The listing builds one solid part. Answer for the finished solid, in the listing's coordinates (mm). A direction names the side the tool comes from. Coordinates: 2 decimals unless noted, no trailing zeros. Order: outer loops, then holes, each group sorted by start corner. A loop starts at its lowest first (then second) coordinate and runs counter-clockwise, first axis right, second up. Notation, with made-up numbers: (22, 53) -> (28, 53) arc R5 ccw to (28, 61) -> close; hole circle Ø4 at (-16, 20). An arc over 180 degrees is marked (long way). Answer in a Markdown table with one row per item. Add a question column.
```python
from build123d import *

# Parameters (mm, degrees)
F0_W     = 119.054884
F0_H     = 68.104512
F1_DEPTH = 25.4
F2_R     = 23.34143
F3_DEPTH = 47.244
F5_DEPTH = 32.512


with BuildPart() as f1:
    # F0 (on Top) → F1 (new body)
    with BuildSketch(Plane.XY):
        Rectangle(F0_W, F0_H)
    extrude(amount=F1_DEPTH)

    # F2 (on face) → F3 (join)
    with BuildSketch(Plane.XY.offset(25.4)):
        Circle(F2_R)
    extrude(amount=F3_DEPTH)

    # F4 (on Front) → F5 (cut, symmetric)
    with BuildSketch(Plane.XZ):
        Polygon((40.58107, 78.345791), (-36.091031, 78.345791), (40.58107, 38.148768), align=None)
    extrude(amount=F5_DEPTH, both=True, mode=Mode.SUBTRACT)


solid = f1.part
```
Q1. Straight lines are drawn through the part: line 1 (Z direction, x = 28, y = -7.5); line 2 (X direction, y = -0.5, z = 30); line 3 (X direction, y = 19.5, z = 32.5). For each, find the intervals that lie inside material, in ascending order.
Q2. Given pin 1 (10 mm diameter, centred on x = 43, y = 21, fed in from +Z); pin 2 (5 mm diameter, centred on x = -7.5, y = 14.5, fed in from -Z); pin 3 (12 mm diameter, centred on y = -14.5, z = 49.5, fed in from +X); pin 4 (12 mm diameter, centred on y = 19, z = 61, fed in from -X), each flat-ended and moving along its own axis, determine where each tip first touches the part or whether it passes through.
Q3. A cutting plane is placed at B-B (x = 0). Determine the outline of the cut face in (y, z), then the cut area to 3 significant figures.
Q4. For faces 1 (the face through (-23.32, 1.03, 43.26)), 2 (the face through (-1, 34.052, 13)), determine the directions among +Z, -Z, +X, -X, +Y, -Y from which every point of the face is accessible in a straight line to the end or side of a thin tool.
Q5. A cutting plane is placed at D-D (x = 38). Determine the outline of the cut face in (y, z), then the cut area to 3 significant figures.
Q6. A cutting plane is placed at C-C (z = 39.5). Determine the outline of the cut face in (x, y).
Q7. A cutting plane is placed at A-A (y = 0). Determine the outline of the cut face in (x, z), then the cut area to 3 significant figures.
Returned:
| question | item | result |
|---|---|---|
| 1 | line 1 | z = 0 to 25.4 |
| 1 | line 2 | x = -23.34 to 23.34 |
| 1 | line 3 | x = -12.83 to 12.83 |
| 2 | pin 1 | stops at z = 25.4 |
| 2 | pin 2 | stops at z = 0 |
| 2 | pin 3 | stops at x = 21.67 |
| 2 | pin 4 | stops at x = -19.39 |
| 3 | outline | (-34.05, 0) -> (34.05, 0) -> (34.05, 25.4) -> (23.34, 25.4) -> (23.34, 59.42) -> (-23.34, 59.42) -> (-23.34, 25.4) -> (-34.05, 25.4) -> close |
| 3 | area | 3,320 mm² |
| 4 | face 1 | +Z |
| 4 | face 2 | +Z, -Z, +X, -X, +Y |
| 5 | outline | (-34.05, 0) -> (34.05, 0) -> (34.05, 25.4) -> (-34.05, 25.4) -> close |
| 5 | area | 1,730 mm² |
| 6 | outline | circle Ø46.68 at (0, 0) |
| 7 | outline | (-59.53, 0) -> (59.53, 0) -> (59.53, 25.4) -> (23.34, 25.4) -> (23.34, 47.19) -> (-23.34, 71.66) -> (-23.34, 25.4) -> (-59.53, 25.4) -> close |
| 7 | area | 4,610 mm² |
